Check sheet for the modelled part. Datum: model origin and axes. Units: mm. Give positions to 0.01 mm unless a question says otherwise; leave off trailing zeros. Loops run counter-clockwise (first coordinate to the right, second up) from the corner with the lowest first, then second, coordinate; pieces in that order, holes last. Notation, with made-up numbers: (41.25, 83.5) - (47.25, 83.5) arc R20 ccw to (47.25, 97.5) - close; hole circle Ø7 at (37, 51.5). An arc over 180 degrees is marked (long way). Use one line per item in the form item = value.
Autodesk Inventor part; units mm, degrees
ref_plane "YZ Plane" through (0, 0, 0) normal (1, 0, 0) x (0, 1, 0)
ref_plane "XZ Plane" through (0, 0, 0) normal (0, 1, 0) x (-1, 0, 0)
ref_plane "XY Plane" through (0, 0, 0) normal (0, 0, 1) x (1, 0, 0)
sketch "Sketch1" plane through (0, 0, 0) normal (0, 0, 1) x (1, 0, 0)
  line L0 (-25, 25) -> (25, 25)
  line L1 (25, 25) -> (25, -25)
  line L2 (25, -25) -> (-25, -25)
  line L3 (-25, -25) -> (-25, 25)
  line L4 (-25, 25) -> (25, -25) construction
  line L5 (25, 25) -> (-25, -25) construction
  circle A0 centre (0, 0) radius 8.5
  line L6 (0, 25) -> (0, -25) construction
  arc A1 (0, 25) -> (0, -25) centre (0, 0) ccw
  point P0 (0, 0)
  point P1 (-25, 0)
  dimension "d0" = 50
  dimension "d1" = 50
  dimension "d14" = 17
extrude "Plate1" add sketch "Sketch1" along normal blind 8 contours L0 L1 L2 A1
equation "\"d2\" = Thickness"
equation "\"BendRadius\" = Thickness"
equation "\"BendReliefWidth\" = Thickness"
equation "\"BendReliefDepth\" = 0.5 * Thickness"
equation "\"CornerReliefSize\" = 4 * Thickness"
equation "\"MinimumRemnant\" = 2 * Thickness"
equation "\"TransitionRadius\" = BendRadius"
equation "\"JacobiRadiusSize\" = BendRadius"
equation "\"GapSize\" = Thickness"
properties part number "PNS-0872 roof ring"
Item 1: Section check C-C on x = -16.5. Record the boundary of the cut face in (y, z), then the cut area to 3 significant figures.
Answer block:
outline = (-18.78, 0) - (18.78, 0) - (18.78, 8) - (-18.78, 8) - close
area = 301 mm2
Item 2: Section check B-B on z = 5.75. Record the boundary of the cut face in (x, y), then the cut area to 3 significant figures.
Answer block:
outline = (0, -25) - (25, -25) - (25, 25) - (0, 25) arc R25 ccw to start; hole circle Ø17 at (0, 0)
area = 2,000 mm2
Item 3: Gauge pin test, flat ends, axial feed: P1, Ø2, axis at x = -4.5, z = 3.5, coming from the -Y side; P2, Ø1.5, axis at y = 3.5, z = 1, coming from the -X side. Record the tip position at first contact, or that the pin passes through.
Answer block:
P1 = -24.75
P2 = -24.85
Item 4: Mould release check, pull along Y, two halves, no side actions. Record for faces 1 (the face through (4.57, -7.167, 3.944)), 2 (the face through (13, -25, 4)), 3 (the face through (-24.994, -0.55, 3.944)): released by +Y, released by -Y, zero draft, split by the parting line, or undercut.
Answer block:
face_1 = undercut
face_2 = released by -Y
face_3 = split by the parting line
Item 5: Thickness scan on L1, parallel to Y at x = 0, z = 3.75; L2, parallel to X at y = 2, z = 7.5; L3, parallel to Y at x = -1.5, z = 2.25. Record the ranges inside material, lowest first.
Answer block:
L1 = -25 to -8.5, 8.5 to 25
L2 = -24.92 to -8.26, 8.26 to 25
L3 = -24.95 to -8.37, 8.37 to 24.95
Item 6: Section check D-D on y = 21.5. Record the boundary of the cut face in (x, z), then the cut area to 3 significant figures.
Answer block:
outline = (-12.76, 0) - (25, 0) - (25, 8) - (-12.76, 8) - close
area = 302 mm2
Item 7: Section check A-A on y = 0. Record the boundary of the cut face in (x, z), then the cut area to 3 significant figures.
Answer block:
outline = (-25, 0) - (-8.5, 0) - (-8.5, 8) - (-25, 8) - close; (8.5, 0) - (25, 0) - (25, 8) - (8.5, 8) - close
area = 264 mm2
